Verification items for the finished model (mm, model axes). Face numbers are marked on the shaded views. A direction names the side the tool comes from. Coordinates: 2 decimals unless noted, no trailing zeros. Order: outer loops, then holes, each group sorted by start corner. A loop starts at its lowest first (then second) coordinate and runs counter-clockwise, first axis right, second up. Notation, with made-up numbers: M 24,38 L 33,38 A17 ccw 33,52 Z; hole C 62,60 d3. An arc over 180 degrees is marked long. Return JSON: item names as keys, results as strings. Group by question number.
1. Set-up check for the marked faces 4 and 5: record each of +Z, -Z, +X, -X, +Y, -Y from which the full face is reachable in a straight line by a thin tool's end or side.
2. Section check C-C, the plane z = 0. Record the cut outline in (x, y), plus the area to 3 significant figures.
3. Section check A-A, the plane x = 25. Record the cut outline in (y, z).
4. Mould release check, pull along Z, two halves, no side actions. Record for the marked faces 1, 2 and 3: +Z half, -Z half, draft (parallel to the pull), parting line (faces both ways), or undercut.
5. Material ranges on line 1 along X through (y, z) = (11.5, 0); line 2 along X through (y, z) = (1.1, 0); line 3 along X through (y, z) = (5.75, 0), recorded low to high.
6. Section check B-B, the plane y = 14.25. Record the cut outline in (x, z).
7. Gauge pin test, flat ends, axial feed: pin 1 (9 mm diameter, centred on x = 23, z = -2.5, fed in from +Y); pin 2 (8 mm diameter, centred on y = 10, z = 1, fed in from +X); pin 3 (4 mm diameter, centred on x = -25, z = 0, fed in from +Y). Record the tip position at first contact, or that the pin passes through.
8. Section check D-D, the plane x = -25. Record the cut outline in (y, z).
```python
from build123d import *

# Parameters (mm, degrees)
SKETCH_1_W          = 70
SKETCH_1_H          = 30
EXTRUDE_1_DEPTH     = 15
FILLET_1_R          = 3
SKETCH_5_R          = 1.75
SKETCH_5_R_2        = 3.4
CUT_EXTRUDE_1_DEPTH = 41.926763859
CUT_EXTRUDE_2_DEPTH = 7.8
SKETCH_7_W          = 30.080931192
SKETCH_7_H          = 35.934517801
CUT_EXTRUDE_4_DEPTH = 11
SKETCH_9_R          = 5.5
CUT_EXTRUDE_5_DEPTH = 2.5


with BuildPart() as part:
    # 草图1 → 凸台-拉伸1 (new body)
    with BuildSketch(Plane(origin=(0, 0, 0), x_dir=(1, 0, 0), z_dir=(0, 1, 0))):
        Rectangle(SKETCH_1_W, SKETCH_1_H)
    extrude(amount=EXTRUDE_1_DEPTH)

    # 圆角1
    fillet_1_edges = [part.edges().sort_by_distance(p)[0] for p in [
        (35, 7.5, 15),
        (-35, 7.5, 15),
        (-35, 7.5, -15),
        (35, 7.5, -15),
    ]]
    fillet(fillet_1_edges, radius=FILLET_1_R)

    # 草图5 → 切除-拉伸1 (cut, through all)
    with BuildSketch(Plane(origin=(0, 15, 0), x_dir=(1, 0, 0), z_dir=(0, 1, 0))):
        with Locations(Location((0, 0, 0), (0, 0, 270))):
            Circle(SKETCH_5_R)
        with Locations(Location((-25, 0, 0), (0, 0, 270))):
            Circle(SKETCH_5_R_2)
        with Locations(Location((25, 0, 0), (0, 0, 270))):
            Circle(SKETCH_5_R_2)
    extrude(amount=-CUT_EXTRUDE_1_DEPTH, mode=Mode.SUBTRACT)

    # 草图6 → 切除-拉伸2 (cut)
    with BuildSketch(Plane.XZ):
        Polygon((0, 3.579571669), (-3.1, 1.789785834), (-3.1, -1.789785834), (0, -3.579571669), (3.1, -1.789785834), (3.1, 1.789785834), align=None)
    extrude(amount=-CUT_EXTRUDE_2_DEPTH, mode=Mode.SUBTRACT)

    # 草图7 → 切除-拉伸4 (cut)
    with BuildSketch(Plane(origin=(0, 15, 0), x_dir=(1, 0, 0), z_dir=(0, 1, 0))):
        with Locations((25.049156013, -1.117442304)):
            Rectangle(SKETCH_7_W, SKETCH_7_H)
    extrude(amount=-CUT_EXTRUDE_4_DEPTH, mode=Mode.SUBTRACT)

    # 草图9 → 切除-拉伸5 (cut)
    with BuildSketch(Plane(origin=(0, 4, 0), x_dir=(1, 0, 0), z_dir=(0, 1, 0))):
        with Locations(Location((25, 0, 0), (0, 0, 270))):
            Circle(SKETCH_9_R)
    extrude(amount=-CUT_EXTRUDE_5_DEPTH, mode=Mode.SUBTRACT)


solid = part.part
```
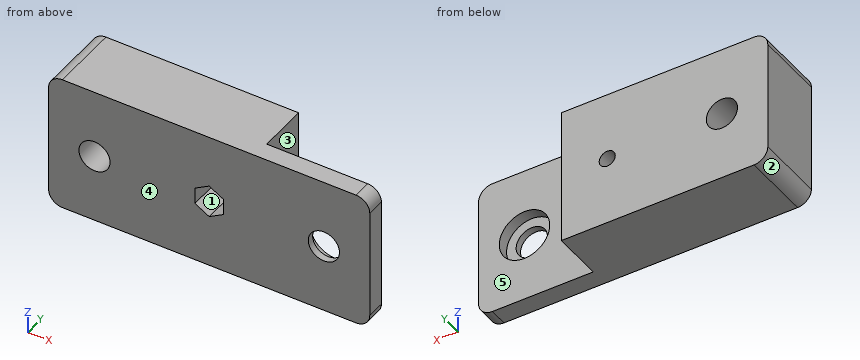
Answers follow:
{
 "1": {"face 4": "+Z, -Z, +X, -X, -Y", "face 5": "+Z, -Z, +X, +Y"},
 "2": {"outline": "M -35,0 L -28.4,0 L -28.4,15 L -35,15 Z; M -21.6,0 L -3.1,0 L -3.1,7.8 L -1.75,7.8 L -1.75,15 L -21.6,15 Z; M 1.75,7.8 L 3.1,7.8 L 3.1,0 L 21.6,0 L 21.6,1.5 L 19.5,1.5 L 19.5,4 L 10.01,4 L 10.01,15 L 1.75,15 Z; M 28.4,0 L 35,0 L 35,4 L 30.5,4 L 30.5,1.5 L 28.4,1.5 Z", "area": "562 mm^2"},
 "3": {"outline": "M 0,-15 L 4,-15 L 4,-5.5 L 1.5,-5.5 L 1.5,-3.4 L 0,-3.4 Z; M 0,3.4 L 1.5,3.4 L 1.5,5.5 L 4,5.5 L 4,15 L 0,15 Z"},
 "4": {"face 1": "undercut", "face 2": "-Z half", "face 3": "draft"},
 "5": {"line 1": "-35 to -28.4, -21.6 to -1.75, 1.75 to 10.01", "line 2": "-35 to -28.4, -21.6 to -3.1, 3.1 to 21.6, 28.4 to 35", "line 3": "-35 to -28.4, -21.6 to -3.1, 3.1 to 10.01"},
 "6": {"outline": "M -35,-12 A3 ccw -32,-15 L 10.01,-15 L 10.01,15 L -32,15 A3 ccw -35,12 Z; hole C -25,0 d6.8; hole C 0,0 d3.5"},
 "7": {"pin 1": "y = 4", "pin 2": "x = 10.01", "pin 3": "through"},
 "8": {"outline": "M 0,-15 L 15,-15 L 15,-3.4 L 0,-3.4 Z; M 0,3.4 L 15,3.4 L 15,15 L 0,15 Z"}
}
